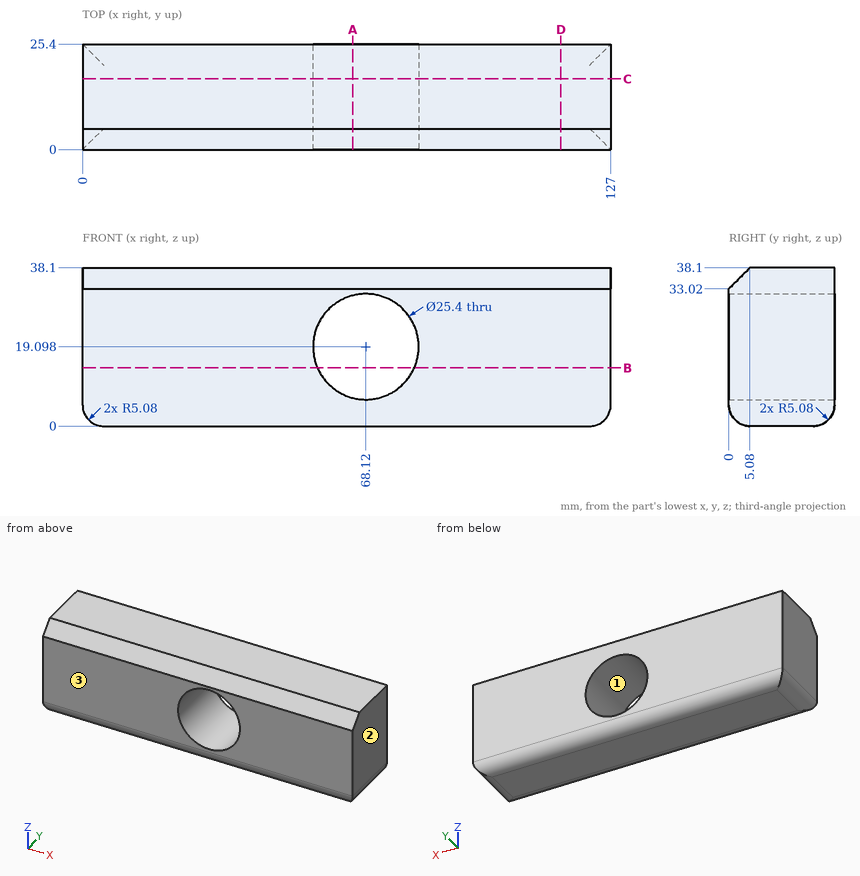
The drawing under review shows one solid part. Ordinate dimensions are in mm from its lowest x, y, z. Round coordinates to 2 decimals unless told otherwise and drop trailing zeros. Write each loop counter-clockwise with the first axis right and the second up, starting at its lowest first coordinate (ties: lowest second). Pieces come first, ordered by that corner, then holes. Notation, with made-up numbers: (-33.75, 9.5) - (25.25, 9.5) arc R31 cw to (25.25, 47.5) - close; hole circle Ø6 at (26, 89). An arc over 180 degrees is marked (long way). Use a Markdown table: item, result. Add a question column.
1. We need section C-C (y = 17). State the section outline as (x, z) points, then the cut area to 3 significant figures.
2. We need section B-B (z = 14). State the section outline as (x, y) points.
3. Wall thickness on probe 1 along Z at (x, y) = (69, 20.5); probe 2 along X at (y, z) = (17, 11.5) (1 decimal); probe 3 along X at (y, z) = (17.25, 19.5): over which ranges is each line inside the solid? List them lowest first.
4. Clearance check with a flat-ended pin moving along its axis: pin 1 (15 mm diameter, centred on x = 68.12, z = 19.1, fed in from -Y). State where the tip first meets the part, or that it passes through.
5. We need section A-A (x = 65). State the section outline as (y, z) points, then the cut area to 3 significant figures.
6. Mouldability with a two-part tool opening along X and no side actions: class the marked faces 1, 2 and 3 as +X half, -X half, draft (parallel to the pull), parting line (faces both ways), or undercut.
7. We need section D-D (x = 115). State the section outline as (y, z) points.
Output:
| question | item | result |
|---|---|---|
| 1 | outline | (0, 5.08) arc R5.08 ccw to (5.08, 0) - (121.92, 0) arc R5.08 ccw to (127, 5.08) - (127, 38.1) - (0, 38.1) - close; hole circle Ø25.4 at (68.12, 19.1) |
| 1 | area | 4,320 mm2 |
| 2 | outline | (0, 0) - (56.49, 0) - (56.49, 25.4) - (0, 25.4) - close; (79.75, 0) - (127, 0) - (127, 25.4) - (79.75, 25.4) - close |
| 3 | probe 1 | z = 0 to 6.43, 31.77 to 38.1 |
| 3 | probe 2 | x = 0 to 57.9, 78.3 to 127 |
| 3 | probe 3 | x = 0 to 55.43, 80.81 to 127 |
| 4 | pin 1 | passes through |
| 5 | outline | (0, 5.08) arc R5.08 ccw to (5.08, 0) - (20.32, 0) arc R5.08 ccw to (25.4, 5.08) - (25.4, 6.79) - (0, 6.79) - close; (0, 31.41) - (25.4, 31.41) - (25.4, 38.1) - (5.08, 38.1) - (0, 33.02) - close |
| 5 | area | 318 mm2 |
| 6 | face 1 | undercut |
| 6 | face 2 | +X half |
| 6 | face 3 | draft |
| 7 | outline | (0, 5.08) arc R5.08 ccw to (5.08, 0) - (20.32, 0) arc R5.08 ccw to (25.4, 5.08) - (25.4, 38.1) - (5.08, 38.1) - (0, 33.02) - close |
